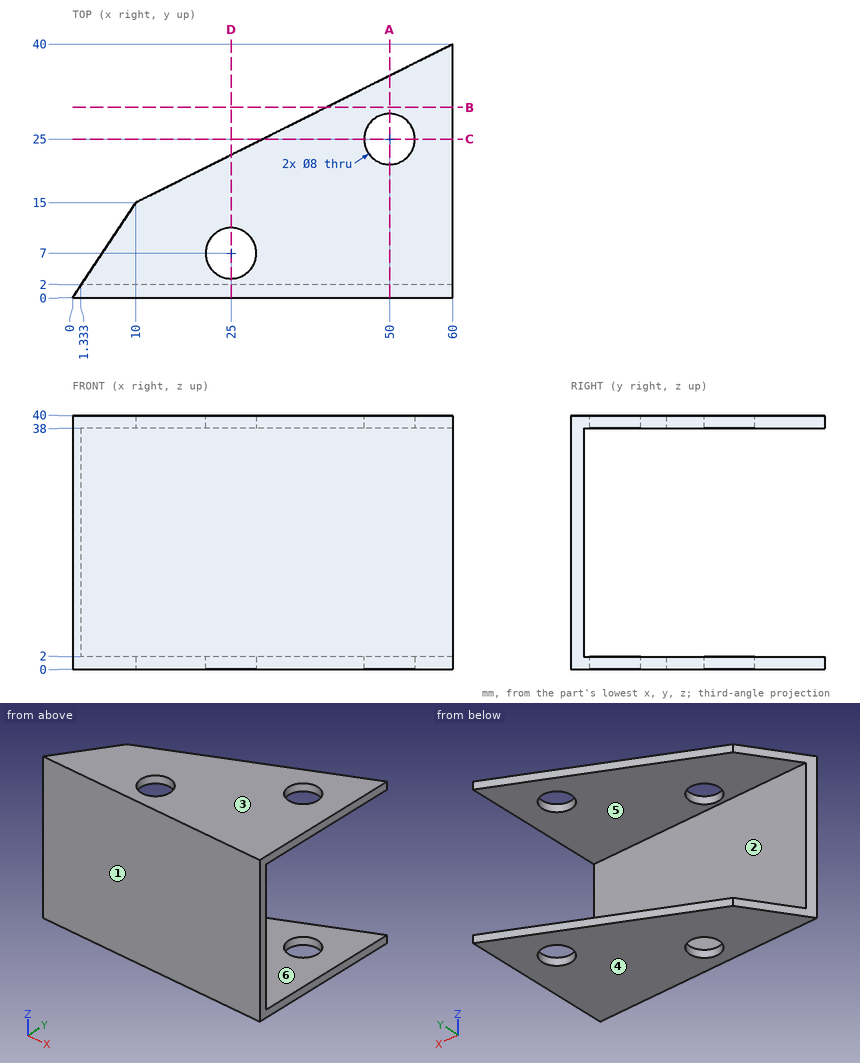
Check sheet for the drawn part. Datum: minimum x, y, z corner. Units: mm. A direction names the side the tool comes from. Round coordinates to 2 decimals unless told otherwise and drop trailing zeros. Write each loop counter-clockwise with the first axis right and the second up, starting at its lowest first coordinate (ties: lowest second). Pieces come first, ordered by that corner, then holes. Notation, with made-up numbers: (56, 42.25) -> (99, 42.25) arc R6 cw to (99, 48.25) -> close; hole circle Ø9 at (88.25, -19). An arc over 180 degrees is marked (long way). Put each result on its own line as item: value.
(1) Tool access check on the marked faces 1 and 2. Record the directions out of +Z, -Z, +X, -X, +Y, -Y that give a thin tool (end or side, any length) a straight path to the whole face; none if there is none.
Values found:
face 1: +Z, -Z, +X, -X, -Y
face 2: +X, -X, +Y
(2) Sectioned sample at B-B (y = 30). Enter the section's corners in (x, z).
Values found:
outline: (40, 0) -> (60, 0) -> (60, 2) -> (40, 2) -> close; (40, 38) -> (60, 38) -> (60, 40) -> (40, 40) -> close
(3) Mould release check, pull along Z, two halves, no side actions. Record for the marked faces 3, 4, 5 and 6: released by +Z, released by -Z, zero draft, split by the parting line, or undercut.
Values found:
face 3: released by +Z
face 4: released by -Z
face 5: undercut
face 6: undercut
(4) Sectioned sample at D-D (x = 25). Enter the section's corners in (y, z).
Values found:
outline: (0, 0) -> (3, 0) -> (3, 2) -> (2, 2) -> (2, 38) -> (3, 38) -> (3, 40) -> (0, 40) -> close; (11, 0) -> (22.5, 0) -> (22.5, 2) -> (11, 2) -> close; (11, 38) -> (22.5, 38) -> (22.5, 40) -> (11, 40) -> close
(5) Material ranges on line 1 (Z direction, x = 6, y = 3); line 2 (Y direction, x = 39.5, z = 12); line 3 (Y direction, x = 25, z = 1), recorded low to high.
Values found:
line 1: z = 0 to 2, 38 to 40
line 2: y = 0 to 2
line 3: y = 0 to 3, 11 to 22.5
(6) Sectioned sample at C-C (y = 25). Enter the section's corners in (x, z).
Values found:
outline: (30, 0) -> (46, 0) -> (46, 2) -> (30, 2) -> close; (30, 38) -> (46, 38) -> (46, 40) -> (30, 40) -> close; (54, 0) -> (60, 0) -> (60, 2) -> (54, 2) -> close; (54, 38) -> (60, 38) -> (60, 40) -> (54, 40) -> close
(7) Sectioned sample at A-A (x = 50). Enter the section's corners in (y, z).
Values found:
outline: (0, 0) -> (21, 0) -> (21, 2) -> (2, 2) -> (2, 38) -> (21, 38) -> (21, 40) -> (0, 40) -> close; (29, 0) -> (35, 0) -> (35, 2) -> (29, 2) -> close; (29, 38) -> (35, 38) -> (35, 40) -> (29, 40) -> close
(8) Go/stop test with a flat-tipped pin: pin 1 Ø3 at (x, z) = (17.5, 17) entering from +Y. Record where the tip stops, or that it passes through.
Values found:
pin 1: stops at y = 2
